Work out the finished part from the listing and answer in its coordinate system (mm). Face numbers are marked on the shaded views. A direction names the side the tool comes from. Coordinates: 2 decimals unless noted, no trailing zeros. Order: outer loops, then holes, each group sorted by start corner. A loop starts at its lowest first (then second) coordinate and runs counter-clockwise, first axis right, second up. Notation, with made-up numbers: (86, 19.25) - (94, 19.25) arc R19 cw to (94, 24.25) - close; hole circle Ø9 at (87.5, 24.5). An arc over 180 degrees is marked (long way). Answer as a JSON object with one key per item and string values. Group by question number.
1) A tool of negligible diameter and unlimited length cuts with its end or side. For the marked faces 4, 5 and 6, from which of +Z, -Z, +X, -X, +Y, -Y can it reach the whole face along a straight path? Write none if from no direction.
2) Section A-A (x = 6) is taken. Give the vertices of the cut face in (y, z), plus the area to 3 significant figures.
3) Section D-D (z = 2.75) is taken. Give the vertices of the cut face in (x, y).
4) The mould has two halves that part along Y. Classify the marked faces 1, 2 and 3: released by +Y, released by -Y, zero draft, split by the parting line, or undercut.
5) Section B-B (y = 5) is taken. Give the vertices of the cut face in (x, z).
6) Section C-C (z = 16.75) is taken. Give the vertices of the cut face in (x, y), plus the area to 3 significant figures.
7) Find the intervals of material crossed by line 1 along Y through (x, z) = (6, 12.5); line 2 along Z through (x, y) = (19.5, 13.25); line 3 along X through (y, z) = (4.5, 12), in increasing order.
8) Each of these flat-tipped pins is pushed along its axis until it touches: P1, Ø1.8, axis at x = 27.64, y = 16.64, coming from the +Z side; P2, Ø5, axis at x = 16.5, z = 13, coming from the +Y side; P3, Ø2, axis at y = 5, z = 8, coming from the +X side; P4, Ø6, axis at x = 22, z = 8.5, coming from the +Y side. Where does it stop, or does it pass through?
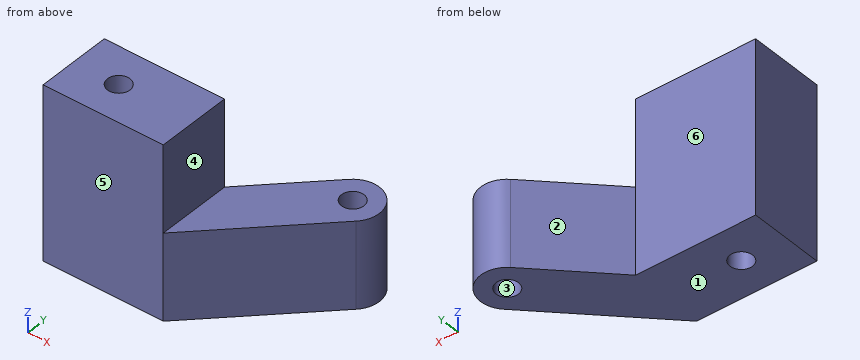
from build123d import *

# Parameters (mm, degrees)
SKETCH_1_R          = 1.5
EXTRUDE_2_DEPTH     = 23
SKETCH_2_W          = 17.071500421
SKETCH_2_H          = 21.570260429
CUT_EXTRUDE_1_DEPTH = 11.5


with BuildPart() as part:
    # 草图1 → 凸台-拉伸2 (new body)
    with BuildSketch(Plane.XY):
        with BuildLine():
            Line((16, 0), (30.142135624, 14.142135624))
            ThreePointArc((30.142135624, 14.142135624), (30.142135624, 19.142135624), (25.142135624, 19.142135624))
            Line((25.142135624, 19.142135624), (16, 10))
            Line((16, 10), (0, 10))
            Line((0, 10), (0, 0))
            Line((0, 0), (16, 0))
        make_face()
        with Locations((27.642135624, 16.642135624)):
            Circle(SKETCH_1_R, mode=Mode.SUBTRACT)
        with Locations((6, 5)):
            Circle(SKETCH_1_R, mode=Mode.SUBTRACT)
    extrude(amount=EXTRUDE_2_DEPTH)

    # 草图2 → 切除-拉伸1 (cut)
    with BuildSketch(Plane.XY.offset(23)):
        with Locations((24.535750211, 10.785130215)):
            Rectangle(SKETCH_2_W, SKETCH_2_H)
    extrude(amount=-CUT_EXTRUDE_1_DEPTH, mode=Mode.SUBTRACT)


solid = part.part
Report:
{
 "1": {"face 4": "+Z, +X, +Y, -Y", "face 5": "+Z, -Z, +X, -X, -Y", "face 6": "+Z, -Z, -X, +Y"},
 "2": {"outline": "(0, 0) - (3.5, 0) - (3.5, 23) - (0, 23) - close; (6.5, 0) - (10, 0) - (10, 23) - (6.5, 23) - close", "area": "161 mm²"},
 "3": {"outline": "(0, 0) - (16, 0) - (30.14, 14.14) arc R3.54 ccw to (25.14, 19.14) - (16, 10) - (0, 10) - close; hole circle Ø3 at (6, 5); hole circle Ø3 at (27.64, 16.64)"},
 "4": {"face 1": "zero draft", "face 2": "released by +Y", "face 3": "undercut"},
 "5": {"outline": "(0, 0) - (4.5, 0) - (4.5, 23) - (0, 23) - close; (7.5, 0) - (21, 0) - (21, 11.5) - (16, 11.5) - (16, 23) - (7.5, 23) - close"},
 "6": {"outline": "(0, 0) - (16, 0) - (16, 10) - (0, 10) - close; hole circle Ø3 at (6, 5)", "area": "153 mm²"},
 "7": {"line 1": "y = 0 to 3.5, 6.5 to 10", "line 2": "z = 0 to 11.5", "line 3": "x = 0 to 4.59, 7.41 to 16"},
 "8": {"P1": "passes through", "P2": "stops at y = 12.5", "P3": "stops at x = 22", "P4": "stops at y = 19"}
}
